Input: part model. Units: mm. Frame: model coordinates. Face numbers are marked on the shaded views. Round coordinates to 2 decimals unless told otherwise and drop trailing zeros. Loops run counter-clockwise (first coordinate to the right, second up) from the corner with the lowest first, then second, coordinate; pieces in that order, holes last. Notation, with made-up numbers: M 6,54.5 L 10,54.5 A16 ccw 10,79.5 Z; hole C -26,-11 d2. An arc over 180 degrees is marked long. Put each result on its own line as item: value. Start each with the question number.
1) Section B-B on y = 0. Output: boundary loops of the cut face in (x, z) (1 decimal).
2) Draft query along X for the marked faces 1, 2 and 3. Return one class per face: +X half, -X half, draft (parallel to the pull), parting line (faces both ways), or undercut.
3) Pin query (flat end, axial travel): pin 1 (20.5 mm diameter, centred on x = 70, y = -70, fed in from +Z); pin 2 (8 mm diameter, centred on x = -7.5, y = -17, fed in from +Z). Return the tip coordinate at first contact, or that it passes through.
4) Section A-A on x = 127. Output: boundary loops of the cut face in (y, z).
5) Section C-C on x = 0. Output: boundary loops of the cut face in (y, z), plus the area to 3 significant figures.
6) Section D-D on z = 18.75. State how many separate pieces and enclosed holes the cut face has, plus the area to 3 significant figures.
7) Line query: probe 1 along X at (y, z) = (-69.5, 19.5) (3 decimals); probe 2 along Y at (x, z) = (-127, 12.25); probe 3 along Y at (x, z) = (0, 24.5). Output: solid intervals per line, ascending.
from build123d import *

# Parameters (mm, degrees)
F0_W     = 285.75
F0_H     = 177.8
F0_R     = 11.43
F0_R_2   = 8.73125
F0_R_3   = 29.9085
F1_DEPTH = 25.4
F0_R_4   = 22.5425
F2_DEPTH = 22.4028
F0_R_5   = 8.128
F3_DEPTH = 15.24
F4_DEPTH = 15.24
F5_DEPTH = 15.24
F6_DEPTH = 15.24


with BuildPart() as f1:
    # F0 (on Top) → F1 (new body)
    with BuildSketch(Plane.XY):
        Rectangle(F0_W, F0_H)
        with Locations((-70.0024, -70.0024)):
            Circle(F0_R, mode=Mode.SUBTRACT)
        with Locations((-127, -34.417)):
            Circle(F0_R_2, mode=Mode.SUBTRACT)
        with Locations((70.0024, -70.0024)):
            Circle(F0_R, mode=Mode.SUBTRACT)
        with Locations((127, -34.417)):
            Circle(F0_R_2, mode=Mode.SUBTRACT)
        with Locations((-127, 34.417)):
            Circle(F0_R_2, mode=Mode.SUBTRACT)
        with Locations((-70.0024, 70.0024)):
            Circle(F0_R, mode=Mode.SUBTRACT)
        Circle(F0_R_3, mode=Mode.SUBTRACT)
        with Locations((127, 34.417)):
            Circle(F0_R_2, mode=Mode.SUBTRACT)
        with Locations((70.0024, 70.0024)):
            Circle(F0_R, mode=Mode.SUBTRACT)
    extrude(amount=F1_DEPTH)

    # F0 (on Top) → F2 (join)
    with BuildSketch(Plane.XY):
        Circle(F0_R_3)
        Circle(F0_R_4, mode=Mode.SUBTRACT)
    extrude(amount=F2_DEPTH)

    # F0 (on Top) → F3 (join)
    with BuildSketch(Plane.XY):
        with Locations((-70.0024, 70.0024)):
            Circle(F0_R)
        with Locations((-70.0024, 70.0024)):
            Circle(F0_R_5, mode=Mode.SUBTRACT)
    extrude(amount=F3_DEPTH)

    # F0 (on Top) → F4 (join)
    with BuildSketch(Plane.XY):
        with Locations((70.0024, 70.0024)):
            Circle(F0_R)
        with Locations((70.0024, 70.0024)):
            Circle(F0_R_5, mode=Mode.SUBTRACT)
    extrude(amount=F4_DEPTH)

    # F0 (on Top) → F5 (join)
    with BuildSketch(Plane.XY):
        with Locations((-70.0024, -70.0024)):
            Circle(F0_R)
        with Locations((-70.0024, -70.0024)):
            Circle(F0_R_5, mode=Mode.SUBTRACT)
    extrude(amount=F5_DEPTH)

    # F0 (on Top) → F6 (join)
    with BuildSketch(Plane.XY):
        with Locations((70.0024, -70.0024)):
            Circle(F0_R)
        with Locations((70.0024, -70.0024)):
            Circle(F0_R_5, mode=Mode.SUBTRACT)
    extrude(amount=F6_DEPTH)


solid = f1.part
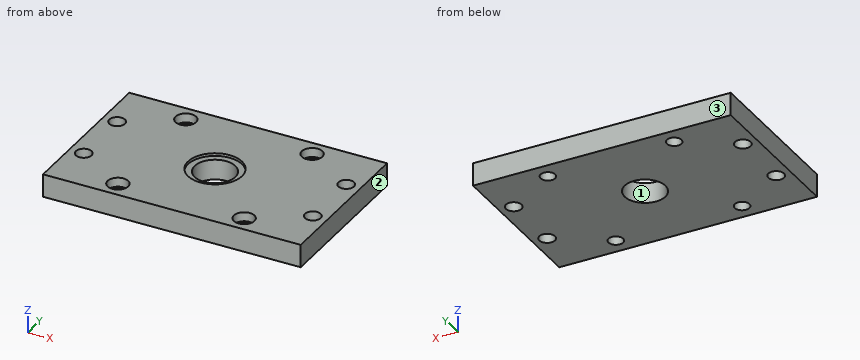
Geometry results:
1. outline: M -142.9,0 L -22.5,0 L -22.5,22.4 L -29.9,22.4 L -29.9,25.4 L -142.9,25.4 Z; M 22.5,0 L 142.9,0 L 142.9,25.4 L 29.9,25.4 L 29.9,22.4 L 22.5,22.4 Z
2. face 1: undercut
2. face 2: +X half
2. face 3: draft
3. pin 1: stops at z = 15.24
3. pin 2: stops at z = 22.4
4. outline: M -88.9,0 L -43.15,0 L -43.15,25.4 L -88.9,25.4 Z; M -25.69,0 L 25.69,0 L 25.69,25.4 L -25.69,25.4 Z; M 43.15,0 L 88.9,0 L 88.9,25.4 L 43.15,25.4 Z
5. outline: M -88.9,0 L -22.54,0 L -22.54,22.4 L -29.91,22.4 L -29.91,25.4 L -88.9,25.4 Z; M 22.54,0 L 88.9,0 L 88.9,25.4 L 29.91,25.4 L 29.91,22.4 L 22.54,22.4 Z
5. area: 3,330 mm²
6. separate pieces: 1
6. enclosed holes: 9
6. area: 46,600 mm²
7. probe 1: x = -142.875 to -81.421, -58.583 to 58.583, 81.421 to 142.875
7. probe 2: y = -88.9 to -43.15, -25.69 to 25.69, 43.15 to 88.9
7. probe 3: y = -88.9 to -29.91, 29.91 to 88.9
